Input: dimensioned drawing with shaded views. Units: mm. Origin: part minimum x, y, z. Give positions to 0.01 mm unless a question says otherwise; leave off trailing zeros. Write each loop counter-clockwise with the first axis right and the second up, starting at its lowest first coordinate (ties: lowest second). Pieces come first, ordered by that corner, then holes.
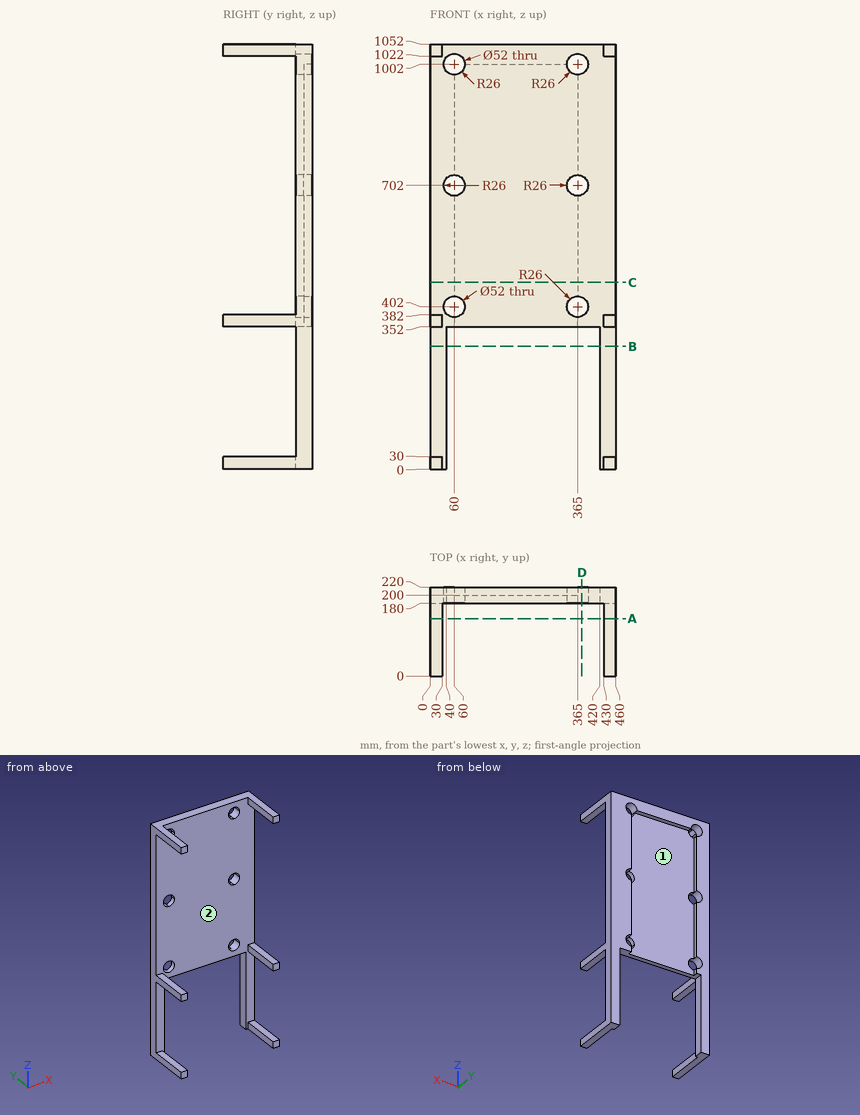
Item 1: Section A-A (y = 142). Return loops of the section in (x, z), and give its area (3 significant figures).
Item 2: Section D-D (x = 376). Return loops of the section in (y, z), and give its area (3 significant figures).
Item 3: Mould query, pull axis Z, two halves, no side actions, for the marked faces 1 and 2. Classes: +Z half, -Z half, draft (parallel to the pull), parting line (faces both ways), or undercut.
Item 4: Section C-C (z = 462). Return loops of the section in (x, y), and give its area (3 significant figures).
Item 5: Section B-B (z = 304). Return loops of the section in (x, y), and give its area (3 significant figures).
Item 6: Pin query (flat end, axial travel): pin 1 (2 mm diameter, centred on x = 266, z = 696, fed in from -Y); pin 2 (6 mm diameter, centred on x = 345.5, z = 487, fed in from +Y). Return the tip coordinate at first contact, or that it passes through.
Item 7: Ray query, line 1 (Z direction, x = 60, y = 194); line 2 (Z direction, x = 434, y = 34.5); line 3 (X direction, y = 198, z = 1002). Return the intervals inside material, ascending.
Solved:
1. outline: (0, 0) - (30, 0) - (30, 30) - (0, 30) - close; (0, 352) - (30, 352) - (30, 382) - (0, 382) - close; (0, 1022) - (30, 1022) - (30, 1052) - (0, 1052) - close; (430, 0) - (460, 0) - (460, 30) - (430, 30) - close; (430, 352) - (460, 352) - (460, 382) - (430, 382) - close; (430, 1022) - (460, 1022) - (460, 1052) - (430, 1052) - close
1. area: 5,400 mm2
2. outline: (180, 352) - (220, 352) - (220, 378.44) - (180, 378.44) - close; (180, 425.56) - (220, 425.56) - (220, 678.44) - (180, 678.44) - close; (180, 725.56) - (220, 725.56) - (220, 978.44) - (180, 978.44) - close; (180, 1025.56) - (220, 1025.56) - (220, 1052) - (180, 1052) - close
2. area: 22,300 mm2
3. face 1: draft
3. face 2: undercut
4. outline: (0, 180) - (460, 180) - (460, 220) - (365, 220) - (365, 200) - (60, 200) - (60, 220) - (0, 220) - close
4. area: 12,300 mm2
5. outline: (0, 180) - (40, 180) - (40, 220) - (0, 220) - close; (420, 180) - (460, 180) - (460, 220) - (420, 220) - close
5. area: 3,200 mm2
6. pin 1: stops at y = 180
6. pin 2: stops at y = 200
7. line 1: z = 352 to 376, 428 to 676, 728 to 976, 1028 to 1052
7. line 2: z = 0 to 30, 352 to 382, 1022 to 1052
7. line 3: x = 0 to 34, 86 to 339, 391 to 460
